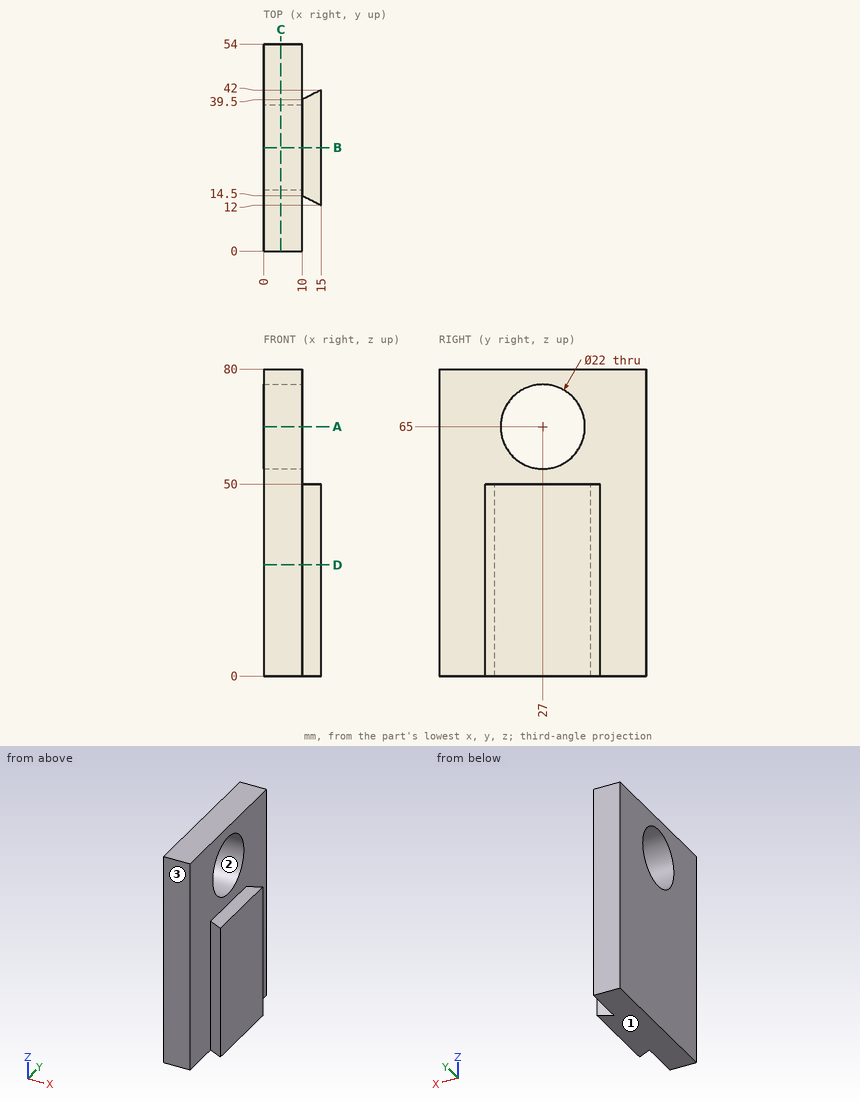
Here's the drawing with two shaded views (mm, measured from the low corner). I have some questions. Coordinates: 2 decimals unless noted, no trailing zeros. Loops run counter-clockwise (first coordinate to the right, second up) from the corner with the lowest first, then second, coordinate; pieces in that order, holes last. Notation, with made-up numbers: M 48.5,-36 L 96.5,-36 A17 ccw 96.5,-3 Z; hole C -23,59 d6. An arc over 180 degrees is marked long. Return JSON: item names as keys, results as strings. Group by question number.
Item 1: I'm going to push flat-ended pins straight in: pin 1 Ø17.5 at (y, z) = (27, 65) entering from -X; pin 2 Ø5.5 at (x, y) = (13, 33) entering from +Z. Where does each tip first touch, or does it pass through?
Item 2: Thinking about a two-plate mould opening in Y: for the marked faces 1, 2 and 3, which applies, released by +Y, released by -Y, zero draft, split by the parting line, or undercut?
Item 3: Imagine slicing it at C-C (x = 4.5). Please give me the cut outline in (y, z).
Item 4: Imagine slicing it at B-B (y = 27). Please give me the cut outline in (x, z).
Item 5: Imagine slicing it at D-D (z = 29). Please give me the cut outline in (x, y), and give its area (4 significant figures).
Item 6: If I drill on L1, parallel to Z at x = 4.75, y = 27; L2, parallel to Z at x = 11, y = 25; L3, parallel to X at y = 47, z = 76.5, over which ranges is the centre line in solid material (lowest first)? Write a range as from..to.
Item 7: Imagine slicing it at A-A (z = 65). Please give me the cut outline in (x, y).
Verdict:
{
 "1": {"pin 1": "passes through", "pin 2": "stops at z = 50"},
 "2": {"face 1": "zero draft", "face 2": "undercut", "face 3": "released by -Y"},
 "3": {"outline": "M 0,0 L 54,0 L 54,80 L 0,80 Z; hole C 27,65 d22"},
 "4": {"outline": "M 0,0 L 15,0 L 15,50 L 10,50 L 10,54 L 0,54 Z; M 0,76 L 10,76 L 10,80 L 0,80 Z"},
 "5": {"outline": "M 0,0 L 10,0 L 10,14.5 L 15,12 L 15,42 L 10,39.5 L 10,54 L 0,54 Z", "area": "677.5 mm^2"},
 "6": {"L1": "z = 0..54, 76..80", "L2": "z = 0..50", "L3": "x = 0..10"},
 "7": {"outline": "M 0,0 L 10,0 L 10,16 L 0,16 Z; M 0,38 L 10,38 L 10,54 L 0,54 Z"}
}
